from build123d import *

# Parameters (mm, degrees)
ESQUISSE1_W             = 42
ESQUISSE1_H             = 20
BOSS_EXTRU_1_DEPTH      = 21
ESQUISSE2_W             = 12
ESQUISSE2_H             = 6
ENL_V_MAT_EXTRU_1_DEPTH = 10
ESQUISSE3_W             = 6
ESQUISSE3_H             = 5
ENL_V_MAT_EXTRU_2_DEPTH = 36.637059362


with BuildPart() as part:
    # Esquisse1 → Boss.-Extru.1 (new body)
    with BuildSketch(Plane(origin=(0, 0, 0), x_dir=(1, 0, 0), z_dir=(0, 1, 0))):
        Rectangle(ESQUISSE1_W, ESQUISSE1_H)
    extrude(amount=BOSS_EXTRU_1_DEPTH)

    # Esquisse2 → Enlèv. mat.-Extru.1 (cut)
    with BuildSketch(Plane(origin=(0, 21, 0), x_dir=(1, 0, 0), z_dir=(0, 1, 0))):
        Rectangle(ESQUISSE2_W, ESQUISSE2_H)
    extrude(amount=-ENL_V_MAT_EXTRU_1_DEPTH, mode=Mode.SUBTRACT)

    # Esquisse3 → Enlèv. mat.-Extru.2 (cut, through all)
    with BuildSketch(Plane(origin=(-6, 0, 0), x_dir=(0, 0, -1), z_dir=(1, 0, 0))):
        with Locations((0, 13.5)):
            Rectangle(ESQUISSE3_W, ESQUISSE3_H)
    extrude(amount=-ENL_V_MAT_EXTRU_2_DEPTH, mode=Mode.SUBTRACT)


solid = part.part
Design review of the part built by this model. Coordinates are the model's own, in mm. A direction names the side the tool comes from. Round coordinates to 2 decimals unless told otherwise and drop trailing zeros. Write each loop counter-clockwise with the first axis right and the second up, starting at its lowest first coordinate (ties: lowest second). Pieces come first, ordered by that corner, then holes.
Item 1: Draft analysis for pull direction Y (two halves, no side actions). For faces 1 (the flat face through (-4, 15, 3)), 2 (the flat face through (21, 10, 0)), 3 (the flat face through (0, 21, -5)), state which applies: released by +Y, released by -Y, zero draft, split by the parting line, or undercut.
Item 2: Consider section B-B on y = 16.75. Give the boundary of the cut face in (x, z), and give its area (3 significant figures).
Item 3: Consider section C-C on x = -16.5. Give the boundary of the cut face in (y, z), and give its area (3 significant figures).
Item 4: Consider section A-A on z = 1. Give the boundary of the cut face in (x, y), and give its area (3 significant figures).
Item 5: Consider section D-D on y = 12.25. Give the boundary of the cut face in (x, z).
Item 6: For faces 4 (the flat face through (-4, 15, -3)), 5 (the flat face through (-7, 11, 0)), 6 (the flat face through (6, 16, 0)), list the 3-axis set-ups (+Z, -Z, +X, -X, +Y, -Y) from which the entire face can be reached by the end or side of a thin tool; tool diameter is ignored.
Item 7: Wall thickness on L1, parallel to Z at x = 1, y = 17; L2, parallel to Y at x = -11, z = -0.5; L3, parallel to X at y = 15.5, z = -2.25: over which ranges is each line inside the solid? List them lowest first.
Check values:
1. face 1: undercut
1. face 2: zero draft
1. face 3: released by +Y
2. outline: (-21, -10) - (21, -10) - (21, 10) - (-21, 10) - close; hole (-6, -3) - (6, -3) - (6, 3) - (-6, 3) - close
2. area: 768 mm2
3. outline: (0, -10) - (21, -10) - (21, 10) - (0, 10) - close; hole (11, -3) - (16, -3) - (16, 3) - (11, 3) - close
3. area: 390 mm2
4. outline: (-21, 0) - (21, 0) - (21, 21) - (6, 21) - (6, 11) - (-21, 11) - close; (-21, 16) - (-6, 16) - (-6, 21) - (-21, 21) - close
4. area: 687 mm2
5. outline: (-21, -10) - (21, -10) - (21, 10) - (-21, 10) - (-21, 3) - (6, 3) - (6, -3) - (-21, -3) - close
6. face 4: none
6. face 5: -X
6. face 6: +Y
7. L1: z = -10 to -3, 3 to 10
7. L2: y = 0 to 11, 16 to 21
7. L3: x = 6 to 21
